Read the model definition and answer for the solid it produces. Units are mm, in the model's axes. A direction names the side the tool comes from. Coordinates: 2 decimals unless noted, no trailing zeros. Loops run counter-clockwise (first coordinate to the right, second up) from the corner with the lowest first, then second, coordinate; pieces in that order, holes last.
from build123d import *

# Parameters (mm, degrees)
SKETCH1_R           = 40
BOSS_EXTRUDE1_DEPTH = 10
SKETCH2_R           = 38
CUT_EXTRUDE1_DEPTH  = 9
CUT_EXTRUDE2_DEPTH  = 8


with BuildPart() as part:
    # Sketch1 → Boss-Extrude1 (new body)
    with BuildSketch(Plane(origin=(0, 0, 0), x_dir=(1, 0, 0), z_dir=(0, 1, 0))):
        with Locations(Location((0, 0, 0), (0, 0, 270))):
            Circle(SKETCH1_R)
    extrude(amount=BOSS_EXTRUDE1_DEPTH)

    # Sketch2 → Cut-Extrude1 (cut)
    with BuildSketch(Plane(origin=(0, 10, 0), x_dir=(1, 0, 0), z_dir=(0, 1, 0))):
        with Locations(Location((0, 0, 0), (0, 0, 270))):
            Circle(SKETCH2_R)
    extrude(amount=-CUT_EXTRUDE1_DEPTH, mode=Mode.SUBTRACT)

    # Sketch4 → Cut-Extrude2 (cut)
    with BuildSketch(Plane.XZ):
        Polygon((-29.11512784, 3.483476928), (-29.11512784, 21.826543334), (-16.809019998, 21.826543334), (-16.809019998, 18.343682624), (-24.47131356, 18.343682624), (-24.47131356, 15.093012628), (-17.50559214, 15.093012628), (-17.50559214, 11.610151918), (-24.47131356, 11.610151918), (-24.47131356, 6.966337638), (-16.809019998, 6.966337638), (-16.809019998, 3.483476928), align=None)
        Polygon((1.766237122, 3.483476928), (-3.537869501, 3.483476928), (-7.140453548, 9.357176396), (-10.811969213, 3.483476928), (-15.880257142, 3.483476928), (-9.651015643, 12.738453669), (-15.648066428, 21.826543334), (-10.347587785, 21.826543334), (-6.973566472, 16.297501957), (-3.534241521, 21.826543334), (1.534046408, 21.826543334), (-4.463004377, 12.919852664), align=None)
        Polygon((12.447009966, 3.483476928), (2.694999978, 3.483476928), (2.694999978, 6.734146924), (5.249097832, 6.734146924), (5.249097832, 18.575873338), (2.694999978, 18.575873338), (2.694999978, 21.826543334), (12.447009966, 21.826543334), (12.447009966, 18.575873338), (9.892912112, 18.575873338), (9.892912112, 6.734146924), (12.447009966, 6.734146924), align=None)
        Polygon((18.948349958, 3.483476928), (18.948349958, 18.343682624), (13.607963536, 18.343682624), (13.607963536, 21.826543334), (28.93255066, 21.826543334), (28.93255066, 18.343682624), (23.592164238, 18.343682624), (23.592164238, 3.483476928), align=None)
        Polygon((-9.246875158, -2.330611882), (-15.552304236, -20.673678288), (-20.355749631, -20.673678288), (-26.661178709, -2.330611882), (-21.995596549, -2.330611882), (-17.957654913, -14.923330137), (-13.912457318, -2.330611882), align=None)
        Polygon((1.433897686, -20.673678288), (-8.318112302, -20.673678288), (-8.318112302, -17.423008292), (-5.764014448, -17.423008292), (-5.764014448, -5.581281878), (-8.318112302, -5.581281878), (-8.318112302, -2.330611882), (1.433897686, -2.330611882), (1.433897686, -5.581281878), (-1.120200168, -5.581281878), (-1.120200168, -17.423008292), (1.433897686, -17.423008292), align=None)
        Polygon((23.027634088, -20.673678288), (18.383819808, -20.673678288), (18.383819808, -8.469153883), (15.147661732, -16.262054722), (12.10015861, -16.262054722), (8.864000534, -8.469153883), (8.864000534, -20.673678288), (4.452376968, -20.673678288), (4.452376968, -2.330611882), (9.807275309, -2.330611882), (13.750889468, -11.32074609), (17.679991706, -2.330611882), (23.027634088, -2.330611882), align=None)
    extrude(amount=-CUT_EXTRUDE2_DEPTH, mode=Mode.SUBTRACT)


solid = part.part
Item 1: A cutting plane is placed at A-A on z = 0. Determine the outline of the cut face in (x, y).
Numbers:
outline: (-40, 0) - (40, 0) - (40, 10) - (38, 10) - (38, 1) - (-38, 1) - (-38, 10) - (-40, 10) - close
Item 2: A cutting plane is placed at C-C on y = 7.75. Determine the outline of the cut face in (x, z), then the cut area to 3 significant figures.
Numbers:
outline: circle Ø80 at (0, 0); hole circle Ø76 at (0, 0)
area: 490 mm2
Item 3: Given pin 1 (0.5 mm diameter, centred on y = 0.5, z = -14, fed in from -X); pin 2 (0.8 mm diameter, centred on y = 0.5, z = 13.5, fed in from -X); pin 3 (0.5 mm diameter, centred on x = -12, y = 0.5, fed in from -Z), each flat-ended and moving along its own axis, determine where each tip first touches the part or whether it passes through.
Numbers:
pin 1: stops at x = -37.56
pin 2: stops at x = -37.79
pin 3: stops at z = -38.24
Item 4: Determine the mould class of faces 4 (the face through (-39.05, 4.93, -8.67)), 5 (the face through (10.505, 0.493, -12.42)), 6 (the face through (1, 0, -1)) for opening direction X: released by +X, released by -X, zero draft, split by the parting line, or undercut.
Numbers:
face 4: split by the parting line
face 5: undercut
face 6: zero draft
Item 5: A cutting plane is placed at B-B on x = 21. Determine the outline of the cut face in (y, z).
Numbers:
outline: (0, -34.04) - (10, -34.04) - (10, -31.67) - (1, -31.67) - (1, -20.67) - (0, -20.67) - close; (0, -2.33) - (1, -2.33) - (1, 3.48) - (0, 3.48) - close; (0, 21.83) - (1, 21.83) - (1, 31.67) - (10, 31.67) - (10, 34.04) - (0, 34.04) - close
Item 6: A cutting plane is placed at D-D on x = 0. Determine the outline of the cut face in (y, z), then the cut area to 3 significant figures.
Numbers:
outline: (0, -40) - (10, -40) - (10, -38) - (1, -38) - (1, -20.67) - (0, -20.67) - close; (0, -17.42) - (1, -17.42) - (1, -5.58) - (0, -5.58) - close; (0, -2.33) - (1, -2.33) - (1, 3.48) - (0, 3.48) - close; (0, 6.16) - (1, 6.16) - (1, 19.55) - (0, 19.55) - close; (0, 21.83) - (1, 21.83) - (1, 38) - (10, 38) - (10, 40) - (0, 40) - close
area: 105 mm2
Item 7: Find the intervals of material crossed by line 1 along X through (y, z) = (5.75, 0); line 2 along X through (y, z) = (9.5, -35); line 3 along Y through (x, z) = (27, -19), in increasing order.
Numbers:
line 1: x = -40 to -38, 38 to 40
line 2: x = -19.36 to -14.8, 14.8 to 19.36
line 3: y = 0 to 1
Item 8: Which of the six approach directions +Z, -Z, +X, -X, +Y, -Y give full straight-line access (tool end or side, diameter ignored) to faces 1 (the face through (-14.6, 10, 35.4)), 2 (the face through (-5.28, 0.49, 19.02)), 3 (the face through (-23.122, 5.563, -30.156))?
Numbers:
face 1: +Z, -Z, +X, -X, +Y
face 2: +Y, -Y
face 3: +Y
